CAD build for the part. Positions are in the model's coordinates, mm. A direction names the side the tool comes from. Round coordinates to 2 decimals unless told otherwise and drop trailing zeros. Loops run counter-clockwise (first coordinate to the right, second up) from the corner with the lowest first, then second, coordinate; pieces in that order, holes last.
```python
from build123d import *

# Parameters (mm, degrees)
SKETCH1_R           = 1.4
BOSS_EXTRUDE1_DEPTH = 2
SKETCH2_W           = 35.6
SKETCH2_H           = 4
BOSS_EXTRUDE2_DEPTH = 2.5
SKETCH3_W           = 35.6
SKETCH3_H           = 2
BOSS_EXTRUDE3_DEPTH = 30
SKETCH4_W           = 3
SKETCH4_H           = 10
BOSS_EXTRUDE4_DEPTH = 2.5
SKETCH5_W           = 35.6
SKETCH5_H           = 2
BOSS_EXTRUDE5_DEPTH = 20
SKETCH6_W           = 29.6
SKETCH6_H           = 4
BOSS_EXTRUDE6_DEPTH = 2.5
SKETCH7_W           = 35.6
SKETCH7_H           = 24.5
BOSS_EXTRUDE7_DEPTH = 4.4
SKETCH8_W           = 29.6
SKETCH8_H           = 2.5
CUT_EXTRUDE1_DEPTH  = 4.4
SKETCH9_W           = 3
SKETCH9_H           = 2.5
CUT_EXTRUDE2_DEPTH  = 4.4
SKETCH10_W          = 35.6
SKETCH10_H          = 20
CUT_EXTRUDE3_DEPTH  = 4.4
SKETCH11_R          = 1.6
CUT_EXTRUDE4_DEPTH  = 10
SKETCH12_W          = 35.6
SKETCH12_H          = 2.5
CUT_EXTRUDE5_DEPTH  = 1
SKETCH13_W          = 35.6
SKETCH13_H          = 10.25
CUT_EXTRUDE6_DEPTH  = 1
SKETCH14_W          = 35.6
SKETCH14_H          = 19
BOSS_EXTRUDE8_DEPTH = 0.05
BOSS_EXTRUDE9_DEPTH = 35.6
SKETCH16_W          = 35.6
SKETCH16_H          = 16.293178749
CUT_EXTRUDE7_DEPTH  = 29
CUT_EXTRUDE8_DEPTH  = 6.2
SKETCH19_W          = 6
SKETCH19_H          = 2.5
CUT_EXTRUDE9_DEPTH  = 29
SKETCH20_W          = 2.8
SKETCH20_H          = 2.8
CUT_EXTRUDE10_DEPTH = 2


with BuildPart() as part:
    # Sketch1 → Boss-Extrude1 (new body)
    with BuildSketch(Plane(origin=(0, 0, 0), x_dir=(1, 0, 0), z_dir=(0, 1, 0))):
        Polygon((-17.8, 3), (17.8, 3), (17.8, -3), (17.8, -7), (-17.8, -7), (-17.8, -3), align=None)
        with Locations(Location((-14.73, 0, 0), (0, 0, 270))):
            Circle(SKETCH1_R, mode=Mode.SUBTRACT)
        with Locations(Location((14.73, 0, 0), (0, 0, 270))):
            Circle(SKETCH1_R, mode=Mode.SUBTRACT)
    extrude(amount=BOSS_EXTRUDE1_DEPTH)

    # Sketch2 → Boss-Extrude2 (add)
    with BuildSketch(Plane(origin=(0, 2, 0), x_dir=(1, 0, 0), z_dir=(0, 1, 0))):
        with Locations((0, -5)):
            Rectangle(SKETCH2_W, SKETCH2_H)
    extrude(amount=BOSS_EXTRUDE2_DEPTH)

    # Sketch3 → Boss-Extrude3 (add)
    with BuildSketch(Plane.XY.offset(7)):
        with Locations((0, 3.5)):
            Rectangle(SKETCH3_W, SKETCH3_H)
    extrude(amount=BOSS_EXTRUDE3_DEPTH)

    # Sketch4 → Boss-Extrude4 (add)
    with BuildSketch(Plane.XZ.offset(-2.5)):
        with Locations((-16.3, 32)):
            Rectangle(SKETCH4_W, SKETCH4_H)
        with Locations((16.3, 32)):
            Rectangle(SKETCH4_W, SKETCH4_H)
    extrude(amount=BOSS_EXTRUDE4_DEPTH)

    # Sketch5 → Boss-Extrude5 (add)
    with BuildSketch(Plane(origin=(0, 4.5, 0), x_dir=(1, 0, 0), z_dir=(0, 1, 0))):
        with Locations((0, -36)):
            Rectangle(SKETCH5_W, SKETCH5_H)
        with Locations((0, -27.75)):
            Rectangle(SKETCH5_W, SKETCH5_H)
    extrude(amount=BOSS_EXTRUDE5_DEPTH)

    # Sketch6 → Boss-Extrude6 (add)
    with BuildSketch(Plane.XZ.offset(-2.5)):
        with Locations((0, 35)):
            Rectangle(SKETCH6_W, SKETCH6_H)
    extrude(amount=BOSS_EXTRUDE6_DEPTH)

    # Sketch7 → Boss-Extrude7 (add)
    with BuildSketch(Plane.XY.offset(37)):
        with Locations((0, 12.25)):
            Rectangle(SKETCH7_W, SKETCH7_H)
    extrude(amount=BOSS_EXTRUDE7_DEPTH)

    # Sketch8 → Cut-Extrude1 (cut)
    with BuildSketch(Plane(origin=(0, 0, 33), x_dir=(-1, 0, 0), z_dir=(0, 0, -1))):
        with Locations((0, 1.25)):
            Rectangle(SKETCH8_W, SKETCH8_H)
    extrude(amount=-CUT_EXTRUDE1_DEPTH, mode=Mode.SUBTRACT)

    # Sketch9 → Cut-Extrude2 (cut)
    with BuildSketch(Plane(origin=(0, 0, 27), x_dir=(-1, 0, 0), z_dir=(0, 0, -1))):
        with Locations((-16.3, 1.25)):
            Rectangle(SKETCH9_W, SKETCH9_H)
        with Locations((16.3, 1.25)):
            Rectangle(SKETCH9_W, SKETCH9_H)
    extrude(amount=-CUT_EXTRUDE2_DEPTH, mode=Mode.SUBTRACT)

    # Sketch10 → Cut-Extrude3 (cut)
    with BuildSketch(Plane.XY.offset(41.4)):
        with Locations((0, 14.5)):
            Rectangle(SKETCH10_W, SKETCH10_H)
    extrude(amount=-CUT_EXTRUDE3_DEPTH, mode=Mode.SUBTRACT)

    # Sketch11 → Cut-Extrude4 (cut)
    with BuildSketch(Plane.XZ):
        with Locations(Location((-14.73, 0, 0), (0, 0, 270))):
            Circle(SKETCH11_R)
        with Locations(Location((14.73, 0, 0), (0, 0, 270))):
            Circle(SKETCH11_R)
    extrude(amount=-CUT_EXTRUDE4_DEPTH, mode=Mode.SUBTRACT)

    # Sketch12 → Cut-Extrude5 (cut)
    with BuildSketch(Plane(origin=(0, 0, 3), x_dir=(-1, 0, 0), z_dir=(0, 0, -1))):
        with Locations((0, 3.25)):
            Rectangle(SKETCH12_W, SKETCH12_H)
    extrude(amount=-CUT_EXTRUDE5_DEPTH, mode=Mode.SUBTRACT)

    # Sketch13 → Cut-Extrude6 (cut)
    with BuildSketch(Plane(origin=(0, 24.5, 0), x_dir=(1, 0, 0), z_dir=(0, 1, 0))):
        with Locations((0, -31.875)):
            Rectangle(SKETCH13_W, SKETCH13_H)
    extrude(amount=-CUT_EXTRUDE6_DEPTH, mode=Mode.SUBTRACT)

    # Sketch14 → Boss-Extrude8 (add)
    with BuildSketch(Plane.XY.offset(28.75)):
        with Locations((0, 14)):
            Rectangle(SKETCH14_W, SKETCH14_H)
    extrude(amount=BOSS_EXTRUDE8_DEPTH)

    # Sketch15 → Boss-Extrude9 (add)
    with BuildSketch(Plane.ZY.offset(17.8)):
        Polygon((35.120614758, 5.184040287), (41.618997482, 23.038200082), (43.498382723, 22.354159795), (37, 4.5), (34.871644455, 4.5), (26.145386721, 4.5), (27.415135268, 7.988605462), (33.913517991, 25.842765257), (35.792903233, 25.15872497), (29.29452051, 7.304565175), align=None)
    extrude(amount=-BOSS_EXTRUDE9_DEPTH)

    # Sketch16 → Cut-Extrude7 (cut)
    with BuildSketch(Plane(origin=(0, -7.876565314, 21.640685344), x_dir=(-1, 0, 0), z_dir=(0, 0.34202014332566366, -0.9396926207859103))):
        with Locations((0, 23.085226048)):
            Rectangle(SKETCH16_W, SKETCH16_H)
    extrude(amount=CUT_EXTRUDE7_DEPTH, mode=Mode.SUBTRACT)


with BuildPart() as body_2:
    # of the pieces the cut leaves, the one that is kept (cut_extrude7_keep)
    add(part.part.solids().sort_by_distance((-17.8, 0, -3))[0])

    # Sketch17 → Cut-Extrude8 (cut)
    with BuildSketch(Plane(origin=(0, -8.560605601, 23.520070585), x_dir=(1, 0, 0), z_dir=(0, -0.34202014332566366, 0.9396926207859103))):
        Polygon((-17.8, 33.565068136), (-17.8, 35.883362097), (17.8, 35.883362097), (17.8, 33.565068136), (17.8, 16.883362097), (-17.8, 16.883362097), align=None)
    extrude(amount=CUT_EXTRUDE8_DEPTH, mode=Mode.SUBTRACT)

    # Sketch19 → Cut-Extrude9 (cut)
    with BuildSketch(Plane.ZY.offset(-14.8)):
        with Locations((34.4, 1.25)):
            Rectangle(SKETCH19_W, SKETCH19_H)
    extrude(amount=-CUT_EXTRUDE9_DEPTH, mode=Mode.SUBTRACT)

    # Sketch20 → Cut-Extrude10 (cut)
    with BuildSketch(Plane.XZ):
        with Locations((-16.4, 40)):
            Rectangle(SKETCH20_W, SKETCH20_H)
    extrude(amount=-CUT_EXTRUDE10_DEPTH, mode=Mode.SUBTRACT)


solid = body_2.part
```
Item 1: Probe line 1 (X direction, y = 0.55, z = 0); line 2 (Y direction, x = -8.5, z = 22); line 3 (Z direction, x = 5.5, y = 22.25). List the from-to ranges inside material, lowest first.
Answers follow:
line 1: x = -17.8 to -16.33, -13.13 to 13.13, 16.33 to 17.8
line 2: y = 2.5 to 4.5
line 3: z = 32.61 to 34.73, 41.33 to 43.46
Item 2: Cut at B-B, the plane z = 0. Give the cut face in (x, y).
Answers follow:
outline: (-17.8, 0) - (-16.33, 0) - (-16.33, 2) - (-17.8, 2) - close; (-13.13, 0) - (13.13, 0) - (13.13, 2) - (-13.13, 2) - close; (16.33, 0) - (17.8, 0) - (17.8, 2) - (16.33, 2) - close
Item 3: Two-plate mould, pull along Z, no slides. Class faces 1 (the flat face through (0, 2, 41.4)), 2 (the cylindrical face through (-16.3, 1, 0.3)), 3 (the flat face through (-16, 2, 40)): released by +Z, released by -Z, zero draft, split by the parting line, or undercut.
Answers follow:
face 1: released by +Z
face 2: undercut
face 3: zero draft
Item 4: Flat gauge pins, fed straight in: P1, Ø3, axis at x = -16.5, z = 39.5, coming from the -Y side; P2, Ø3, axis at y = 6.5, z = 22.5, coming from the -X side; P3, Ø4, axis at x = 14.73, z = 0, coming from the +Y side; P4, Ø7.5, axis at x = -5.5, z = 1.5, coming from the +Y side. Where does each tip first touch, or does it go through?
Answers follow:
P1: stops at y = 0
P2: passes through
P3: stops at y = 2
P4: stops at y = 4.5
Item 5: Cut at A-A, the plane x = 14.73. Give the cut face in (y, z).
Answers follow:
outline: (0, -3) - (2, -3) - (2, -1.6) - (0, -1.6) - close; (0, 1.6) - (2, 1.6) - (2, 4) - (4.5, 4) - (4.5, 26.15) - (25.84, 33.91) - (25.16, 35.79) - (7.3, 29.29) - (5.18, 35.12) - (23.04, 41.62) - (22.35, 43.5) - (4.5, 37) - (4.5, 41.4) - (0, 41.4) - (0, 37.4) - (2.5, 37.4) - (2.5, 7) - (0, 7) - close
Item 6: Cut at C-C, the plane y = 21. Give the cut face in (x, z).
Answers follow:
outline: (-17.8, 32.15) - (17.8, 32.15) - (17.8, 34.28) - (-17.8, 34.28) - close; (-17.8, 40.88) - (17.8, 40.88) - (17.8, 43.01) - (-17.8, 43.01) - close
Item 7: Cut at D-D, the plane x = 7.5. Give the cut face in (y, z).
Answers follow:
outline: (0, -3) - (2, -3) - (2, 4) - (4.5, 4) - (4.5, 26.15) - (25.84, 33.91) - (25.16, 35.79) - (7.3, 29.29) - (5.18, 35.12) - (23.04, 41.62) - (22.35, 43.5) - (4.5, 37) - (4.5, 41.4) - (0, 41.4) - (0, 37.4) - (2.5, 37.4) - (2.5, 7) - (0, 7) - close
Item 8: 3-axis set-ups, long thin cutter, end or side, ignore diameter. For faces 4 (the flat face through (-0.249, 13.552, 40.295)), 5 (the flat face through (-16, 1, 31.4)), 6 (the flat face through (-14.8, 1, 34)), 7 (the flat face through (0, 2, 0)): which of +Z, -Z, +X, -X, +Y, -Y reach the whole face in a straight line?
Answers follow:
face 4: +Z, +X, -X
face 5: +X, -X, -Y
face 6: +X, -Y
face 7: -Z, +X, -X, +Y
